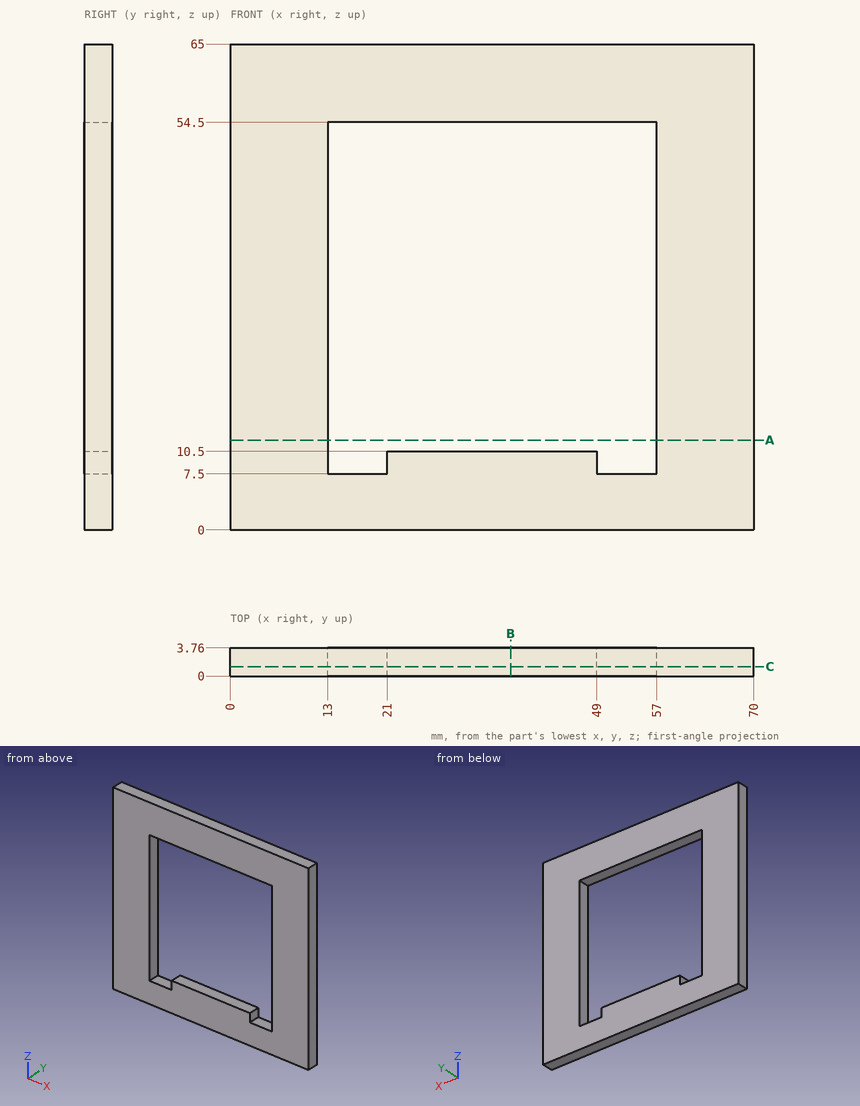
Here's the drawing with two shaded views (mm, measured from the low corner). I have some questions. Give positions to 0.01 mm unless a question says otherwise; leave off trailing zeros. Write each loop counter-clockwise with the first axis right and the second up, starting at its lowest first coordinate (ties: lowest second). Pieces come first, ordered by that corner, then holes. Notation, with made-up numbers: (24.25, -5) -> (42.25, -5) arc R26 cw to (42.25, 18) -> close; hole circle Ø3 at (36, 87). An arc over 180 degrees is marked (long way). Answer as a JSON object with one key per item and string values. Group by question number.
Item 1: Suppose I cut it at C-C (y = 1.25). Please give me the cut outline in (x, z).
Item 2: Please list where these lines run through material, in increasing order: line 1 (X direction, y = 0.85, z = 18.5); line 2 (Z direction, x = 54, y = 0.45); line 3 (Z direction, x = 27.5, y = 2.7). Write a range as [from, to].
Item 3: Suppose I cut it at B-B (x = 37.5). Please give me the cut outline in (y, z), plus the area to 3 significant figures.
Item 4: Suppose I cut it at A-A (z = 12). Please give me the cut outline in (x, y).
Findings:
{
 "1": {"outline": "(0, 0) -> (70, 0) -> (70, 65) -> (0, 65) -> close; hole (13, 7.5) -> (21, 7.5) -> (21, 10.5) -> (49, 10.5) -> (49, 7.5) -> (57, 7.5) -> (57, 54.5) -> (13, 54.5) -> close"},
 "2": {"line 1": "x = [0, 13], [57, 70]", "line 2": "z = [0, 7.5], [54.5, 65]", "line 3": "z = [0, 10.5], [54.5, 65]"},
 "3": {"outline": "(0, 0) -> (3.76, 0) -> (3.76, 10.5) -> (0, 10.5) -> close; (0, 54.5) -> (3.76, 54.5) -> (3.76, 65) -> (0, 65) -> close", "area": "79.0 mm²"},
 "4": {"outline": "(0, 0) -> (13, 0) -> (13, 3.76) -> (0, 3.76) -> close; (57, 0) -> (70, 0) -> (70, 3.76) -> (57, 3.76) -> close"}
}
